```python
from build123d import *

# Parameters (mm, degrees)
F0_W      = 15
F0_H      = 13
F0_R      = 2.5
F1_DEPTH  = 5
F2_W      = 28
F2_H      = 13
F3_DEPTH  = 29
F5_DEPTH  = 13.001
F6_W      = 25
F6_H      = 5
F7_DEPTH  = 1
F9_DEPTH  = 14
F10_R     = 12
F11_DEPTH = 2.65
F12_R     = 12
F13_DEPTH = 2.65
F14_R     = 5.925
F15_DEPTH = 4
F16_R     = 4
F17_DEPTH = 14.351
F19_SIZE  = 3
F21_DEPTH = 5
F23_DEPTH = 5
F24_W     = 25
F24_H     = 3
F25_DEPTH = 1
F27_DEPTH = 1.65
F29_DEPTH = 1.65
F30_W     = 10
F30_H     = 8.3
F31_DEPTH = 3


with BuildPart() as f1:
    # F0 (on Top) → F1 (new body)
    with BuildSketch(Plane.XY):
        with Locations((-20, 0)):
            Rectangle(F0_W, F0_H)
        with Locations((-21, 0)):
            Circle(F0_R, mode=Mode.SUBTRACT)
    extrude(amount=F1_DEPTH)


with BuildPart() as f1b:
    # F0 (on Top) → F1, piece 2 (new body)
    with BuildSketch(Plane.XY):
        with Locations((20, 0)):
            Rectangle(F0_W, F0_H)
        with Locations((21, 0)):
            Circle(F0_R, mode=Mode.SUBTRACT)
    extrude(amount=F1_DEPTH)


with BuildPart() as f3:
    # F2 (on Top) → F3 (new body)
    with BuildSketch(Plane.XY):
        Rectangle(F2_W, F2_H)
    extrude(amount=F3_DEPTH)

    # F4 (on face) → F5 (cut, through all)
    with BuildSketch(Plane.XZ.offset(6.5)):
        with BuildLine():
            ThreePointArc((-14, 15), (-9.8994949366, 24.8994949366), (0, 29))
            Line((0, 29), (-14, 29))
            Line((-14, 29), (-14, 15))
        make_face()
        with BuildLine():
            ThreePointArc((0, 29), (9.8994949366, 24.8994949366), (14, 15))
            Line((14, 15), (14, 29))
            Line((14, 29), (0, 29))
        make_face()
    extrude(amount=-F5_DEPTH, mode=Mode.SUBTRACT)

    # F6 (on face) → F7 (cut)
    with BuildSketch(Plane(origin=(0, 0, 0), x_dir=(1, 0, 0), z_dir=(0, 0, -1))):
        with Locations((0, 4)):
            Rectangle(F6_W, F6_H)
        with Locations((0, -4)):
            Rectangle(F6_W, F6_H)
    extrude(amount=-F7_DEPTH, mode=Mode.SUBTRACT)

    # F8 (on Right) → F9 (cut, symmetric)
    with BuildSketch(Plane.YZ):
        Polygon((-6.5, 29), (-6.5, 5), (-4.85, 15), (-4.85, 29), align=None)
        Polygon((4.85, 29), (4.85, 15), (6.5, 5), (6.5, 29), align=None)
    extrude(amount=F9_DEPTH, both=True, mode=Mode.SUBTRACT)

    # F10 (on face) → F11 (cut)
    with BuildSketch(Plane.XZ.offset(6.5)):
        with Locations((0, 15)):
            Circle(F10_R)
    extrude(amount=-F11_DEPTH, mode=Mode.SUBTRACT)

    # F12 (on face) → F13 (cut)
    with BuildSketch(Plane(origin=(0, 6.5, 0), x_dir=(-1, 0, 0), z_dir=(0, 1, 0))):
        with Locations((0, 15)):
            Circle(F12_R)
    extrude(amount=-F13_DEPTH, mode=Mode.SUBTRACT)

    # F14 (on face) → F15 (join)
    with BuildSketch(Plane.XZ.offset(3.85)):
        with Locations((0, 15)):
            Circle(F14_R)
    extrude(amount=F15_DEPTH)

    # F16 (on face) → F17 (cut, through all)
    with BuildSketch(Plane.XZ.offset(7.85)):
        with Locations((0, 15)):
            Circle(F16_R)
    extrude(amount=-F17_DEPTH, mode=Mode.SUBTRACT)


with BuildPart() as f1_1:
    add(f1.part)

    # F18: union F3, F1b
    add(f3.part)
    add(f1b.part)

    # F19
    f19_edges = [f1_1.edges().sort_by_distance(p)[0] for p in [
        (27.5, -6.5, 2.5),
        (27.5, 6.5, 2.5),
        (-27.5, -6.5, 2.5),
        (-27.5, 6.5, 2.5),
    ]]
    chamfer(f19_edges, length=F19_SIZE)

    # F20 (on face) → F21 (cut)
    with BuildSketch(Plane.XZ.offset(6.5)):
        with BuildLine():
            ThreePointArc((12.5, 8.6952398935), (7.3393922678, 3.0780319938), (-6.31e-08, 1))
            Line((-6.31e-08, 1), (12.5, 1))
            Line((12.5, 1), (12.5, 8.6952398935))
        make_face()
        with BuildLine():
            ThreePointArc((-6.31e-08, 1), (-7.3393923215, 3.0780320269), (-12.5, 8.6952398935))
            Line((-12.5, 8.6952398935), (-12.5, 1))
            Line((-12.5, 1), (-6.31e-08, 1))
        make_face()
    extrude(amount=-F21_DEPTH, mode=Mode.SUBTRACT)

    # F22 (on face) → F23 (cut)
    with BuildSketch(Plane(origin=(0, 6.5, 0), x_dir=(-1, 0, 0), z_dir=(0, 1, 0))):
        with BuildLine():
            ThreePointArc((12.5, 8.6952398935), (7.3393922574, 3.0780319875), (-8.75e-08, 1))
            Line((-8.75e-08, 1), (12.5, 1))
            Line((12.5, 1), (12.5, 8.6952398935))
        make_face()
        with BuildLine():
            ThreePointArc((-8.75e-08, 1), (-7.3393923319, 3.0780320333), (-12.5, 8.6952398935))
            Line((-12.5, 8.6952398935), (-12.5, 1))
            Line((-12.5, 1), (-8.75e-08, 1))
        make_face()
    extrude(amount=-F23_DEPTH, mode=Mode.SUBTRACT)

    # F24 (on face) → F25 (cut)
    with BuildSketch(Plane(origin=(0, 0, 0), x_dir=(1, 0, 0), z_dir=(0, 0, -1))):
        Rectangle(F24_W, F24_H)
    extrude(amount=-F25_DEPTH, mode=Mode.SUBTRACT)

    # F26 (on face) → F27 (cut)
    with BuildSketch(Plane.XZ.offset(6.5)):
        with BuildLine():
            ThreePointArc((-12.5, 8.6952398935), (-11.3010372549, 6.7364319472), (-9.7979589711, 5))
            ThreePointArc((-9.7979589711, 5), (0, 1), (9.7979589711, 5))
            ThreePointArc((9.7979589711, 5), (11.3010372549, 6.7364319472), (12.5, 8.6952398935))
            Line((12.5, 8.6952398935), (12, 15))
            ThreePointArc((12, 15), (10.5735281474, 9.3254513381), (6.6332495807, 5))
            ThreePointArc((6.6332495807, 5), (0, 3), (-6.6332495807, 5))
            ThreePointArc((-6.6332495807, 5), (-10.5735281474, 9.3254513381), (-12, 15))
            Line((-12, 15), (-12.5, 8.6952398935))
        make_face()
    extrude(amount=-F27_DEPTH, mode=Mode.SUBTRACT)

    # F28 (on face) → F29 (cut)
    with BuildSketch(Plane(origin=(0, 6.5, 0), x_dir=(-1, 0, 0), z_dir=(0, 1, 0))):
        with BuildLine():
            Line((-12, 15), (-12.5, 8.6952398935))
            ThreePointArc((-12.5, 8.6952398935), (-11.3010372549, 6.7364319472), (-9.7979589711, 5))
            ThreePointArc((-9.7979589711, 5), (0, 1), (9.7979589711, 5))
            ThreePointArc((9.7979589711, 5), (11.3010372549, 6.7364319472), (12.5, 8.6952398935))
            Line((12.5, 8.6952398935), (12, 15))
            ThreePointArc((12, 15), (10.5735281474, 9.3254513381), (6.6332495807, 5))
            ThreePointArc((6.6332495807, 5), (0, 3), (-6.6332495807, 5))
            ThreePointArc((-6.6332495807, 5), (-10.5735281474, 9.3254513381), (-12, 15))
        make_face()
    extrude(amount=-F29_DEPTH, mode=Mode.SUBTRACT)

    # F30 (on face) → F31 (cut)
    with BuildSketch(Plane(origin=(0, 0, 0), x_dir=(1, 0, 0), z_dir=(0, 0, -1))):
        with Locations((-20, 0)):
            Rectangle(F30_W, F30_H)
        with Locations((20, 0)):
            Rectangle(F30_W, F30_H)
    extrude(amount=-F31_DEPTH, mode=Mode.SUBTRACT)


solid = f1_1.part
```
Can you work these out from the model? Positions are in its coordinate system, mm. A direction names the side the tool comes from. Round coordinates to 2 decimals unless told otherwise and drop trailing zeros. Order: outer loops, then holes, each group sorted by start corner. A loop starts at its lowest first (then second) coordinate and runs counter-clockwise, first axis right, second up.
(1) If we section it at C-C (z = 18): Please give me the cut outline in (x, y).
Results are:
outline: (-13.67, -4.85) - (-11.62, -4.85) - (-11.62, -3.85) - (-5.11, -3.85) - (-5.11, -7.85) - (-2.65, -7.85) - (-2.65, 3.85) - (-11.62, 3.85) - (-11.62, 4.85) - (-13.67, 4.85) - close; (2.65, -7.85) - (5.11, -7.85) - (5.11, -3.85) - (11.62, -3.85) - (11.62, -4.85) - (13.67, -4.85) - (13.67, 4.85) - (11.62, 4.85) - (11.62, 3.85) - (2.65, 3.85) - close
(2) We'd pull the mould along X, two halves only. Please class faces 1 (the face through (-15, 0, 1)), 2 (the face through (13.208, -5.687, 9.93)), 3 (the face through (27.5, 0, 2)): +X half, -X half, draft (parallel to the pull), parting line (faces both ways), or undercut.
Results are:
face 1: undercut
face 2: draft
face 3: +X half
(3) If I drill on L1, parallel to X at y = 0, z = 4.25; L2, parallel to X at y = 4.6, z = 15; L3, parallel to Z at x = 0, y = -3.75, over which ranges is the centre line in solid material (lowest first)?
Results are:
L1: x = -27.5 to -23.5, -18.5 to 18.5, 23.5 to 27.5
L2: x = -14 to -12, 12 to 14
L3: z = 1 to 11, 19 to 29
(4) I'm going to push flat-ended pins straight in: pin 1 (12 mm diameter, centred on x = 3, z = 12.5, fed in from +Y); pin 2 (12 mm diameter, centred on x = 6, z = 19.5, fed in from -Y); pin 3 (6 mm diameter, centred on x = 3.5, z = 4.5, fed in from -Y); pin 4 (4 mm diameter, centred on x = -0.5, z = 6.5, fed in from -Y). Where does each tip first touch, or does it pass through?
Results are:
pin 1: stops at y = 3.85
pin 2: stops at y = -7.85
pin 3: stops at y = -4.85
pin 4: stops at y = -3.85
(5) If we section it at B-B (z = 3.75): Count the separate pieces of the cut face and the enclosed holes in it, plus the area to 3 significant figures.
Results are:
separate pieces: 1
enclosed holes: 2
area: 503 mm2
(6) On a 3-axis mill with a long thin cutter (end or side, diameter ignored), from which of +Z, -Z, +X, -X, +Y, -Y can I reach the whole of each face in a straight line? I mean faces 4 (the face through (0, 0, 1)), 5 (the face through (-0.1, -4.85, 2.8)), 6 (the face through (-0.1, -4.85, 27.2)), 7 (the face through (-18, 0, 3)), 8 (the face through (3, 3.85, 18)). Say none if no direction works.
Results are:
face 4: -Z, +Y, -Y
face 5: -Z, -Y
face 6: +Z, -Y
face 7: -Z
face 8: +Y
(7) If we section it at A-A (x = 21): Please give me the cut outline in (y, z).
Results are:
outline: (-6.5, 0) - (-4.15, 0) - (-4.15, 3) - (-2.5, 3) - (-2.5, 5) - (-6.5, 5) - close; (2.5, 3) - (4.15, 3) - (4.15, 0) - (6.5, 0) - (6.5, 5) - (2.5, 5) - close
(8) If we section it at D-D (z = 22): Please give me the cut outline in (x, y), plus the area to 3 significant figures.
Results are:
outline: (-12.12, -4.85) - (-9.75, -4.85) - (-9.75, -3.85) - (9.75, -3.85) - (9.75, -4.85) - (12.12, -4.85) - (12.12, 4.85) - (9.75, 4.85) - (9.75, 3.85) - (-9.75, 3.85) - (-9.75, 4.85) - (-12.12, 4.85) - close
area: 196 mm2
